CAD build for the part. Positions are in the model's coordinates, mm. A direction names the side the tool comes from. Give positions to 0.01 mm unless a question says otherwise; leave off trailing zeros. Order: outer loops, then holes, each group sorted by start corner. A loop starts at its lowest first (then second) coordinate and runs counter-clockwise, first axis right, second up. Notation, with made-up numbers: M -4.5,-11 L 26.5,-11 A27 ccw 26.5,24 Z; hole C 78,-18 d6. An arc over 180 degrees is marked long. Put each result on its own line as item: value. Start each with the question number.
1) Cut at B-B (z = 0). Write the cut outline in (x, y), and give its area (3 significant figures).
2) Pin check, flat tips, straight feed: pin 1 (1 mm diameter, centred on x = 13.5, y = -21.5, fed in from -Z); pin 2 (5 mm diameter, centred on x = -1, y = -5, fed in from +Z); pin 3 (2 mm diameter, centred on y = -3, z = -2, fed in from +X). Stop position of each tip, or through.
3) Two-plate mould, pull along X, no slides. Class faces 1 (the face through (15, -45, 0)), 2 (the face through (-11.5, -29, 0.1)): released by +X, released by -X, zero draft, split by the parting line, or undercut.
4) Cut at A-A (y = -16). Write the cut outline in (x, z).
5) Tool access for faces 3 (the face through (-14, -45, 0)), 4 (the face through (11.5, -29.5, 0.1)): list every direction of +Z, -Z, +X, -X, +Y, -Y with a clear straight run to the whole face (end or side of a thin tool).
6) Drill centre lines: line 1 (X direction, y = -17.5, z = 2.25); line 2 (X direction, y = -34, z = 1); line 3 (Y direction, x = 6, z = -2). Where is each one in solid material? Low to high. Write a range as [from, to].
Autodesk Inventor part; units mm, degrees
ref_plane "YZ Plane" through (0, 0, 0) normal (1, 0, 0) x (0, 1, 0)
ref_plane "XZ Plane" through (0, 0, 0) normal (0, 1, 0) x (-1, 0, 0)
ref_plane "XY Plane" through (0, 0, 0) normal (0, 0, 1) x (1, 0, 0)
sketch "Náčrt5" plane through (0, 0, 0) normal (1, 0, 0) x (0, 1, 0)
  circle A0 centre (0, 0) radius 3
  dimension "d23" = 6
sketch "Náčrt6" plane through (0, 0, 0) normal (0, 0, 1) x (1, 0, 0)
  line L0 (-14.5, -45) -> (-14.5, -14.5)
  line L1 (0, 0) -> (0, 0)
  line L2 (14.5, -14.5) -> (14.5, -45)
  line L3 (-14.5, -45) -> (14.5, -45) construction
  arc A0 (0, 0) -> (-14.5, -14.5) centre (0, -14.5) ccw
  arc A1 (14.5, -14.5) -> (0, 0) centre (0, -14.5) ccw
  point P0 (0, 0)
  point P1 (14.5, 0)
  point P2 (0, 0)
  dimension "d46" = 29
  dimension "d47" = 45
  dimension "d48" = 14.5
sweep "Tažení4" add profiles "Náčrt5" path "Náčrt6"
chamfer "Zkosení4" distance 1 angle 45 5 edges at (-11.5, -45, 0) (-11.5, -14.5, 0) (0, -3, 0) (11.5, -14.5, 0) (11.5, -45, 0)
equation "\"d48\" = 0.5 * d46"
properties part number "DD_KVD_002_14" material "Nerezová ocel"
Solution:
1. outline: M -17.5,-44 L -16.5,-45 L -12.5,-45 L -11.5,-44 L -11.5,-14.5 A11.5 cw 11.5,-14.5 L 11.5,-44 L 12.5,-45 L 16.5,-45 L 17.5,-44 L 17.5,-14.5 A17.5 ccw -17.5,-14.5 Z
1. area: 637 mm²
2. pin 1: z = -2.96
2. pin 2: z = 1.73
2. pin 3: x = 13.41
3. face 1: zero draft
3. face 2: undercut
4. outline: C -14.5,0 d6; C 14.5,0 d6
5. face 3: +Z, -Z, +X, -X, -Y
5. face 4: -Y
6. line 1: [-16.48, -12.52], [12.52, 16.48]
6. line 2: [-17.33, -11.67], [11.67, 17.33]
6. line 3: [-3.8, 1.12]
